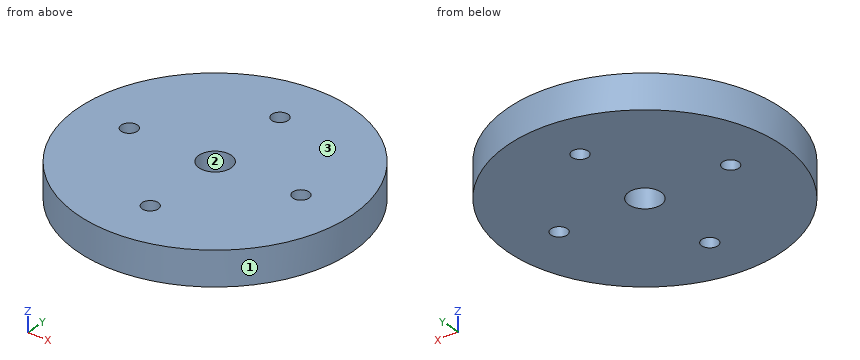
Autodesk Fusion 360 part; units mm, degrees
sketch "Sketch1" plane through (0, 0, 0) normal (0, 0, 1) x (1, 0, 0)
  circle A0 centre (0, 0) radius 50.8
  line L0 (0, 0) -> (0, 31.75) construction
  circle A1 centre (0, 31.75) radius 3
  circle A2 centre (-31.75, 0) radius 3
  circle A3 centre (0, -31.75) radius 3
  circle A4 centre (31.75, 0) radius 3
  circle A5 centre (0, 0) radius 6
  dimension "d1" = 101.6
  dimension "d2" = 31.75
  dimension "d3" = 6
  dimension "d5" = 360
  dimension "d6" = 12
extrude "Extrude1" add sketch "Sketch1" along normal blind 12.7
sketch "Sketch2" plane through (0, 0, 12.7) normal (0, 0, 1) x (-1, 0, 0)
  circle A0 centre (0, -31.75) radius 3
  circle A1 centre (31.75, 0) radius 3
  circle A2 centre (0, 31.75) radius 3
  circle A3 centre (-31.75, 0) radius 3
  circle A4 centre (0, 0) radius 6
  circle A5 centre (0, 0) radius 50.8
equation "d2 = 2.5 in / 2"
Can you work these out from the model? Positions are in its coordinate system, mm. Face numbers are marked on the shaded views. Give positions to 0.01 mm unless a question says otherwise; leave off trailing zeros. Write each loop counter-clockwise with the first axis right and the second up, starting at its lowest first coordinate (ties: lowest second). Pieces come first, ordered by that corner, then holes. Notation, with made-up numbers: M 80.25,1.5 L 114.25,1.5 A27 cw 114.25,37.5 Z; hole C -39,11.5 d7. An arc over 180 degrees is marked long. Answer in a Markdown table with one row per item. Add a question column.
Item 1: Please list where these lines run through material, in increasing order: L1, parallel to Y at x = 0, z = 8.25; L2, parallel to X at y = 1, z = 5.5; L3, parallel to Y at x = 31.75, z = 9.
Item 2: We'd pull the mould along X, two halves only. Please class the marked faces 1, 2 and 3: released by +X, released by -X, zero draft, split by the parting line, or undercut.
Item 3: For pin 1 Ø3 at (x, z) = (-10, 5.5) entering from +Y; pin 2 Ø6 at (y, z) = (-17.5, 4.5) entering from +X; pin 3 Ø3 at (y, z) = (27, 5.5) entering from -X; pin 4 Ø11 at (x, y) = (0, 0) entering from +Z, each with a flat end and sliding along its axis, tell me the tip position at first contact or that it passes through.
Item 4: Imagine slicing it at A-A, the plane x = 0. Write out the boundary of the cut face in (y, z).
Item 5: Imagine slicing it at B-B, the plane y = -31.75. Write out the boundary of the cut face in (x, z), plus the area to 3 significant figures.
Item 6: Imagine slicing it at C-C, the plane z = 6.25. Write out the boundary of the cut face in (x, y).
Evaluation:
| question | item | result |
|---|---|---|
| 1 | L1 | y = -50.8 to -34.75, -28.75 to -6, 6 to 28.75, 34.75 to 50.8 |
| 1 | L2 | x = -50.79 to -34.58, -28.92 to -5.92, 5.92 to 28.92, 34.58 to 50.79 |
| 1 | L3 | y = -39.66 to -3, 3 to 39.66 |
| 2 | face 1 | split by the parting line |
| 2 | face 2 | undercut |
| 2 | face 3 | zero draft |
| 3 | pin 1 | stops at y = 50.08 |
| 3 | pin 2 | stops at x = 48.69 |
| 3 | pin 3 | stops at x = -43.94 |
| 3 | pin 4 | passes through |
| 4 | outline | M -50.8,0 L -34.75,0 L -34.75,12.7 L -50.8,12.7 Z; M -28.75,0 L -6,0 L -6,12.7 L -28.75,12.7 Z; M 6,0 L 28.75,0 L 28.75,12.7 L 6,12.7 Z; M 34.75,0 L 50.8,0 L 50.8,12.7 L 34.75,12.7 Z |
| 5 | outline | M -39.66,0 L -3,0 L -3,12.7 L -39.66,12.7 Z; M 3,0 L 39.66,0 L 39.66,12.7 L 3,12.7 Z |
| 5 | area | 931 mm² |
| 6 | outline | C 0,0 d101.6; hole C -31.75,0 d6; hole C 0,0 d12; hole C 0,-31.75 d6; hole C 0,31.75 d6; hole C 31.75,0 d6 |
